from build123d import *

# Parameters (mm, degrees)
F1_DEPTH = 127
F2_W     = 8.0518
F2_H     = 2.3876
F2_H_2   = 99.2124
F3_DEPTH = 138.90725
F5_DEPTH = 4.7635
F6_R     = 4.365625
F7_DEPTH = 149.3403


# Not quite as in the source:
# - a feature names something its author has since deleted; it is built from what else it names


with BuildPart() as f1:
    # F0 (on Front) → F1 (new body)
    with BuildSketch(Plane.XZ):
        with BuildLine():
            ThreePointArc((-8.0518, 8.0518), (-5.6934823808, 2.3583176192), (0, 0))
            Line((0, 0), (141.2875, 0))
            Line((141.2875, 0), (141.2875, 4.7625))
            Line((141.2875, 4.7625), (0, 4.7625))
            ThreePointArc((0, 4.7625), (-2.3258863354, 5.7259136646), (-3.2893, 8.0518))
            Line((-3.2893, 8.0518), (-3.2893, 138.90625))
            Line((-3.2893, 138.90625), (-8.0518, 138.90625))
            Line((-8.0518, 138.90625), (-8.0518, 8.0518))
        make_face()
    extrude(amount=-F1_DEPTH)

    # F2 (on face) → F3 (cut, through all)
    with BuildSketch(Plane.XY.offset(138.90625)):
        with Locations((-4.0259, 125.8062)):
            Rectangle(F2_W, F2_H)
        with Locations((-4.0259, 49.6062)):
            Rectangle(F2_W, F2_H_2)
    extrude(amount=-F3_DEPTH, mode=Mode.SUBTRACT)

    # F4 (on face) → F5 (cut, through all)
    with BuildSketch(Plane.XY.offset(4.7625)):
        with BuildLine():
            Line((44.45, 90.090625), (57.15, 90.090625))
            ThreePointArc((57.15, 90.090625), (60.721875, 93.6625), (57.15, 97.234375))
            Line((57.15, 97.234375), (44.45, 97.234375))
            ThreePointArc((44.45, 97.234375), (40.878125, 93.6625), (44.45, 90.090625))
        make_face()
        with BuildLine():
            Line((96.8380470509, 115.4906250419), (109.5212624401, 115.490625))
            ThreePointArc((109.5212624401, 115.490625), (113.0931374401, 119.0625055472), (109.5212513457, 122.634375))
            Line((109.5212513457, 122.634375), (96.8212513457, 122.6343355532))
            ThreePointArc((96.8212513457, 122.6343355532), (93.2493862179, 119.0540626774), (96.8380470509, 115.4906250419))
        make_face()
        with BuildLine():
            Line((44.4505470509, 29.7656250419), (57.0326853587, 29.7675520605))
            Line((57.0326853587, 29.7675520605), (57.2684081472, 29.7675881627))
            ThreePointArc((57.2684081472, 29.7675881627), (60.7213841756, 33.3967122102), (57.15, 36.909375))
            Line((57.15, 36.909375), (44.45, 36.909375))
            ThreePointArc((44.45, 36.909375), (40.8781250105, 33.3372264746), (44.4505470509, 29.7656250419))
        make_face()
        with BuildLine():
            Line((141.2875, 127), (128.5875, 127))
            ThreePointArc((128.5875, 127), (137.5677561211, 123.2802561211), (141.2875, 114.3))
            Line((141.2875, 114.3), (141.2875, 127))
        make_face()
        with BuildLine():
            ThreePointArc((6.35, 19.05), (1.8598719395, 20.9098719395), (0, 25.4))
            Line((0, 25.4), (0, 0))
            Line((0, 0), (63.5, 0))
            ThreePointArc((63.5, 0), (59.0098719395, 1.8598719395), (57.15, 6.35))
            Line((57.15, 6.35), (57.15, 19.05))
            Line((57.15, 19.05), (6.35, 19.05))
        make_face()
        with BuildLine():
            ThreePointArc((28.575, 111.9124), (25.4, 115.0874), (22.225, 111.9124))
            ThreePointArc((22.225, 111.9124), (25.4, 108.7374), (28.575, 111.9124))
        make_face()
        with BuildLine():
            Line((96.8380470509, 4.3656250419), (109.5212624401, 4.365625))
            ThreePointArc((109.5212624401, 4.365625), (113.0931374401, 7.9375055472), (109.5212513457, 11.509375))
            Line((109.5212513457, 11.509375), (96.8212513457, 11.5093355532))
            ThreePointArc((96.8212513457, 11.5093355532), (93.2493862179, 7.9290626774), (96.8380470509, 4.3656250419))
        make_face()
        with BuildLine():
            Line((141.2875, 0), (141.2875, 12.7))
            ThreePointArc((141.2875, 12.7), (137.5677561211, 3.7197438789), (128.5875, 0))
            Line((128.5875, 0), (141.2875, 0))
        make_face()
    extrude(amount=-F5_DEPTH, mode=Mode.SUBTRACT)

    # F6 (on face) → F7 (cut, through all)
    with BuildSketch(Plane(origin=(-8.0518, 0, 0), x_dir=(0, -1, 0), z_dir=(-1, 0, 0))):
        with BuildLine():
            Line((-121.4374, 105.56875), (-124.6124, 105.56875))
            Line((-124.6124, 105.56875), (-124.6124, 96.0440792053))
            Line((-124.6124, 96.0440792053), (-121.4933961759, 96.0440792053))
            Line((-121.4933961759, 96.0440792053), (-121.3814038241, 96.0440792053))
            ThreePointArc((-121.3814038241, 96.0440792053), (-116.674982302, 100.8342485718), (-121.4374, 105.56875))
        make_face()
        with Locations((-111.9124, 129.38125)):
            Circle(F6_R)
        with Locations((-111.9124, 73.81875)):
            Circle(F6_R)
    extrude(amount=-F7_DEPTH, mode=Mode.SUBTRACT)


solid = f1.part
Could you check a few things on this model? Use its own coordinates, in mm. A direction names the side the tool comes from. Round coordinates to 2 decimals unless told otherwise and drop trailing zeros. Order: outer loops, then holes, each group sorted by start corner. A loop starts at its lowest first (then second) coordinate and runs counter-clockwise, first axis right, second up.
(1) Imagine slicing it at B-B (z = 12.5). Write out the boundary of the cut face in (x, y), plus the area to 3 significant figures.
Response values:
outline: (-8.05, 99.21) - (-3.29, 99.21) - (-3.29, 124.61) - (-8.05, 124.61) - close
area: 121 mm2
(2) Imagine slicing it at C-C (y = 15). Write out the boundary of the cut face in (x, z), plus the area to 3 significant figures.
Response values:
outline: (57.15, 0) - (141.29, 0) - (141.29, 4.76) - (57.15, 4.76) - close
area: 401 mm2
(3) Please list where these lines run through material, in increasing order: line 1 along Y through (x, z) = (25.4, 3.15); line 2 along Z through (x, y) = (121.5, 13).
Response values:
line 1: y = 19.05 to 108.74, 115.09 to 127
line 2: z = 0 to 4.76
(4) Imagine slicing it at A-A (x = 25.4). Write out the boundary of the cut face in (y, z).
Response values:
outline: (19.05, 0) - (108.74, 0) - (108.74, 4.76) - (19.05, 4.76) - close; (115.09, 0) - (127, 0) - (127, 4.76) - (115.09, 4.76) - close
(5) I'm going to push flat-ended pins straight in: pin 1 (4 mm diameter, centred on x = 12.5, y = 99.5, fed in from +Z); pin 2 (9 mm diameter, centred on x = -4.5, z = 66.5, fed in from -Y); pin 3 (2.5 mm diameter, centred on x = 51.5, z = 2, fed in from -Y); pin 4 (1 mm diameter, centred on x = 25.5, y = 100.5, fed in from -Z). Where does each tip first touch, or does it pass through?
Response values:
pin 1: stops at z = 4.76
pin 2: stops at y = 99.21
pin 3: stops at y = 19.05
pin 4: stops at z = 0
(6) Which directions (+Z, -Z, +X, -X, +Y, -Y) give clear straight access to the entire face, cutting with the end or side of a thin tool? Please do faces 5 (the flat face through (57.15, 13, 2)), 6 (the flat face through (-3.289, 106, 73)), 7 (the cylindrical face through (113.092, 118.984, 2.415)).
Response values:
face 5: +Z, -Z, -X, -Y
face 6: +Z, +X, +Y, -Y
face 7: +Z, -Z
(7) If we mould it in two halves opening along Y, with no side actions, what happens to faces 1 (the flat face through (141.288, 63, 2)), 2 (the flat face through (96, 0, 2)), 3 (the cylindrical face through (40.88, 93.74, 2.41)), 4 (the flat face through (51, 97.234, 2))? For each: released by +Y, released by -Y, zero draft, split by the parting line, or undercut.
Response values:
face 1: zero draft
face 2: released by -Y
face 3: undercut
face 4: undercut
